from build123d import *

# Parameters (mm, degrees)
F0_W     = 76
F0_H     = 27
F0_W_2   = 60
F0_H_2   = 14.8
F1_DEPTH = 3
F2_SIZE  = 2.8
F3_SIZE  = 1.8


with BuildPart() as f1:
    # F0 (on Top) → F1 (new body)
    with BuildSketch(Plane.XY):
        Rectangle(F0_W, F0_H)
        Rectangle(F0_W_2, F0_H_2, mode=Mode.SUBTRACT)
    extrude(amount=F1_DEPTH)

    # F2
    f2_edges = [f1.edges().sort_by_distance(p)[0] for p in [
        (0, 7.4, 3),
        (30, 0, 3),
        (0, -7.4, 3),
        (-30, 0, 3),
    ]]
    chamfer(f2_edges, length=F2_SIZE)

    # F3
    f3_edges = [f1.edges().sort_by_distance(p)[0] for p in [
        (0, 13.5, 3),
        (-38, 0, 3),
        (0, -13.5, 3),
        (38, 0, 3),
    ]]
    chamfer(f3_edges, length=F3_SIZE)


solid = f1.part
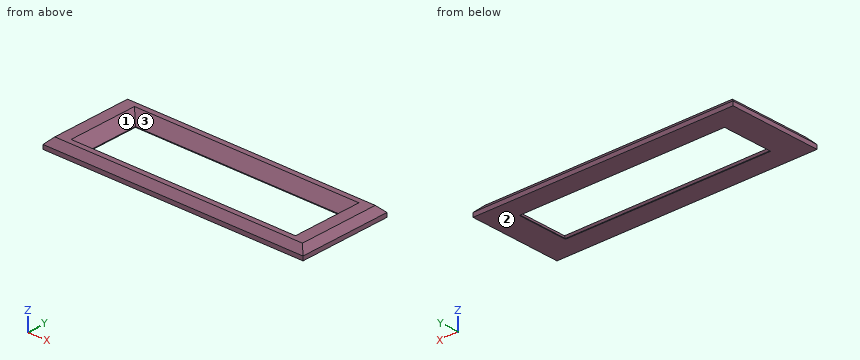
Could you check a few things on this model? Use its own coordinates, in mm. Face numbers are marked on the shaded views. Give positions to 0.01 mm unless a question says otherwise; leave off trailing zeros. Order: outer loops, then holes, each group sorted by start corner. A loop starts at its lowest first (then second) coordinate and runs counter-clockwise, first axis right, second up. Notation, with made-up numbers: (6.5, 58) - (36.5, 58) arc R25 ccw to (36.5, 86) - close; hole circle Ø8 at (7.5, 77). An arc over 180 degrees is marked (long way). One line per question, with ' | ' between items. Start each with the question number.
Item 1: I need wall thicknesses on probe 1 along X at (y, z) = (6, 0.35); probe 2 along X at (y, z) = (-7, 0.5); probe 3 along Y at (x, z) = (23, 2.25). Which ranges of each line are inside material? Lowest first, please. Write a range as [from, to].
Item 2: I want a section at D-D on y = 8.75. Write out the boundary of the cut face in (x, z).
Item 3: I want a section at A-A on x = 21.5. Write out the boundary of the cut face in (y, z).
Item 4: Thinking about a two-plate mould opening in Y: for the marked faces 1, 2 and 3, which applies, pulls with the +Y half, pulls with the -Y half, needs draft (parallel to the pull), parting line crosses it, or undercut?
Item 5: I want a section at C-C on z = 2.15. Write out the boundary of the cut face in (x, y).
Item 6: I want a section at B-B on y = -2. Write out the boundary of the cut face in (x, z), then the cut area to 3 significant figures.
Verdict:
1) probe 1: [-38, -30.15], [30.15, 38] | probe 2: [-38, -30.3], [30.3, 38] | probe 3: [-12.45, -9.45], [9.45, 12.45]
2) outline: (-38, 0) - (38, 0) - (38, 1.2) - (36.2, 3) - (32.8, 3) - (31.35, 1.55) - (-31.35, 1.55) - (-32.8, 3) - (-36.2, 3) - (-38, 1.2) - close
3) outline: (-13.5, 0) - (-7.4, 0) - (-7.4, 0.2) - (-10.2, 3) - (-11.7, 3) - (-13.5, 1.2) - close; (7.4, 0) - (13.5, 0) - (13.5, 1.2) - (11.7, 3) - (10.2, 3) - (7.4, 0.2) - close
4) face 1: undercut | face 2: needs draft | face 3: undercut
5) outline: (-37.05, -12.55) - (37.05, -12.55) - (37.05, 12.55) - (-37.05, 12.55) - close; hole (-31.95, -9.35) - (31.95, -9.35) - (31.95, 9.35) - (-31.95, 9.35) - close
6) outline: (-38, 0) - (-30, 0) - (-30, 0.2) - (-32.8, 3) - (-36.2, 3) - (-38, 1.2) - close; (30, 0) - (38, 0) - (38, 1.2) - (36.2, 3) - (32.8, 3) - (30, 0.2) - close | area: 36.9 mm^2
